Verification items for the finished model (mm, model axes). A direction names the side the tool comes from. Give positions to 0.01 mm unless a question says otherwise; leave off trailing zeros. Write each loop counter-clockwise with the first axis right and the second up, starting at its lowest first coordinate (ties: lowest second). Pieces come first, ordered by that corner, then holes.
from build123d import *

# Parameters (mm, degrees)
SKETCH_1_W          = 50
SKETCH_1_H          = 20
EXTRUDE_3_DEPTH     = 3
SKETCH_2_R          = 5
SKETCH_2_W          = 30
SKETCH_2_H          = 10
CUT_EXTRUDE_1_DEPTH = 3
SKETCH_3_W          = 30
SKETCH_3_H          = 3
CUT_EXTRUDE_2_DEPTH = 1.5
EXTRUDE_4_REACH     = 43.34
SKETCH_5_W          = 30
SKETCH_5_H          = 3
CUT_EXTRUDE_3_DEPTH = 1.5
EXTRUDE_5_REACH     = 43.34


with BuildPart() as part:
    # 스케치1 → 보스-돌출3 (new body)
    with BuildSketch(Plane.XY):
        Rectangle(SKETCH_1_W, SKETCH_1_H)
    extrude(amount=EXTRUDE_3_DEPTH)

    # 스케치2 → 컷-돌출1 (cut)
    with BuildSketch(Plane.XY.offset(3)):
        with Locations((-15, 0)):
            Circle(SKETCH_2_R)
        with Locations((15, 0)):
            Circle(SKETCH_2_R)
        Rectangle(SKETCH_2_W, SKETCH_2_H)
    extrude(amount=-CUT_EXTRUDE_1_DEPTH, mode=Mode.SUBTRACT)

    # 스케치3 → 컷-돌출2 (cut)
    with BuildSketch(Plane.XZ.offset(-5)):
        with Locations((0, 1.5)):
            Rectangle(SKETCH_3_W, SKETCH_3_H)
    extrude(amount=-CUT_EXTRUDE_2_DEPTH, mode=Mode.SUBTRACT)

    # 스케치4 → 보스-돌출4 (add, up to next)
    with BuildSketch(Plane(origin=(-15, 0, 0), x_dir=(0, 0, -1), z_dir=(1, 0, 0)), mode=Mode.PRIVATE) as extrude_4_sk1:
        Polygon((-3, 6.5), (-3, 5), (-1.5, 6.5), align=None)
    extrude_4_tool1 = extrude(extrude_4_sk1.sketch, amount=EXTRUDE_4_REACH, mode=Mode.PRIVATE) - part.part
    # 스케치4 → 보스-돌출4 (add, up to next)
    with BuildSketch(Plane(origin=(-15, 0, 0), x_dir=(0, 0, -1), z_dir=(1, 0, 0)), mode=Mode.PRIVATE) as extrude_4_sk2:
        Polygon((0, 6.5), (-1.5, 6.5), (0, 5), align=None)
    extrude_4_tool2 = extrude(extrude_4_sk2.sketch, amount=EXTRUDE_4_REACH, mode=Mode.PRIVATE) - part.part
    add(extrude_4_tool1.solids().sort_by_distance((-15, 6, 2.5))[0])
    add(extrude_4_tool2.solids().sort_by_distance((-15, 6, 0.5))[0])

    # 스케치5 → 컷-돌출3 (cut)
    with BuildSketch(Plane(origin=(0, -5, 0), x_dir=(1, 0, 0), z_dir=(0, 1, 0))):
        with Locations((0, -1.5)):
            Rectangle(SKETCH_5_W, SKETCH_5_H)
    extrude(amount=-CUT_EXTRUDE_3_DEPTH, mode=Mode.SUBTRACT)

    # 스케치6 → 보스-돌출5 (add, up to next)
    with BuildSketch(Plane(origin=(-15, 0, 0), x_dir=(0, 0, -1), z_dir=(1, 0, 0)), mode=Mode.PRIVATE) as extrude_5_sk1:
        Polygon((-1.5, -6.5), (-3, -5), (-3, -6.5), align=None)
    extrude_5_tool1 = extrude(extrude_5_sk1.sketch, amount=EXTRUDE_5_REACH, mode=Mode.PRIVATE) - part.part
    # 스케치6 → 보스-돌출5 (add, up to next)
    with BuildSketch(Plane(origin=(-15, 0, 0), x_dir=(0, 0, -1), z_dir=(1, 0, 0)), mode=Mode.PRIVATE) as extrude_5_sk2:
        Polygon((0, -5), (-1.5, -6.5), (0, -6.5), align=None)
    extrude_5_tool2 = extrude(extrude_5_sk2.sketch, amount=EXTRUDE_5_REACH, mode=Mode.PRIVATE) - part.part
    add(extrude_5_tool1.solids().sort_by_distance((-15, -6, 2.5))[0])
    add(extrude_5_tool2.solids().sort_by_distance((-15, -6, 0.5))[0])


solid = part.part
Item 1: Sectioned sample at A-A on x = -5. Record the cut outline in (y, z).
Answer key:
outline: (-10, 0) - (-5, 0) - (-6.5, 1.5) - (-5, 3) - (-10, 3) - close; (5, 0) - (10, 0) - (10, 3) - (5, 3) - (6.5, 1.5) - close
Item 2: Scan lines: line 1 along X through (y, z) = (0, 0.3); line 2 along X through (y, z) = (-1.5, 1.9); line 3 along Y through (x, z) = (-5.5, 1.25). Record each from-to range of solid material in increasing order.
Answer key:
line 1: x = -25 to -20, 20 to 25
line 2: x = -25 to -19.77, 19.77 to 25
line 3: y = -10 to -6.25, 6.25 to 10
Item 3: Sectioned sample at C-C on z = 0.9. Record the cut outline in (x, y), then the cut area to 3 significant figures.
Answer key:
outline: (-25, -10) - (25, -10) - (25, 10) - (-25, 10) - close; hole (-15, -5.9) - (15, -5.9) - (15, -5) arc R5 ccw to (15, 5) - (15, 5.9) - (-15, 5.9) - (-15, 5) arc R5 ccw to (-15, -5) - close
area: 567 mm2
Item 4: Sectioned sample at B-B on y = 0. Record the cut outline in (x, z), then the cut area to 3 significant figures.
Answer key:
outline: (-25, 0) - (-20, 0) - (-20, 3) - (-25, 3) - close; (20, 0) - (25, 0) - (25, 3) - (20, 3) - close
area: 30.0 mm2
Item 5: Release check for a two-part mould opening along Y. For faces 1 (the face through (0, 7, 3)), 2 (the face through (20, 0, 2)), 3 (the face through (0, 10, 1)) record: released by +Y, released by -Y, zero draft, split by the parting line, or undercut.
Answer key:
face 1: zero draft
face 2: undercut
face 3: released by +Y
Item 6: Set-up check for faces 4 (the face through (15, 5.6, 1.5)), 5 (the face through (-20, 0, 2)), 6 (the face through (-25, 0, 1)): record each of +Z, -Z, +X, -X, +Y, -Y from which the full face is reachable in a straight line by a thin tool's end or side.
Answer key:
face 4: none
face 5: +Z, -Z
face 6: +Z, -Z, -X, +Y, -Y
Item 7: Sectioned sample at D-D on y = -5.75. Record the cut outline in (x, z), then the cut area to 3 significant figures.
Answer key:
outline: (-25, 0) - (25, 0) - (25, 3) - (-25, 3) - close; hole (-15, 0.75) - (15, 0.75) - (15, 2.25) - (-15, 2.25) - close
area: 105 mm2
